Source: CAD feature listing. Evaluate the final solid. Frame: model axes, mm. Face numbers are marked on the shaded views. A direction names the side the tool comes from. Round coordinates to 2 decimals unless told otherwise and drop trailing zeros. Order: outer loops, then holes, each group sorted by start corner. A loop starts at its lowest first (then second) coordinate and runs counter-clockwise, first axis right, second up. Notation, with made-up numbers: (23, 46) -> (43, 46) arc R14 ccw to (43, 68) -> close; hole circle Ø1 at (-10.75, 49). An arc over 180 degrees is marked (long way). Answer as CSV lines item,"result". Start each with the question number.
(1) Contact query for flat-ended pins moving along their axis: P1, Ø5, axis at y = 141, z = 1, coming from the +X side; P2, Ø1.6, axis at x = 20.5, y = 112, coming from the +Z side; P3, Ø5.5, axis at y = 110, z = 0, coming from the +X side; P4, Ø1.6, axis at x = 21.5, y = 121.5, coming from the -Z side. Output: stop coordinate, or through.
(2) Line query: line 1 along Y through (x, z) = (22.2, 0); line 2 along Y through (x, z) = (21.9, 0); line 3 along Z through (x, y) = (21.8, 110). Output: solid intervals per line, ascending. Write a range as from..to.
(3) Section query A-A (z = 0). Count the separate pieces of the cut face and the enclosed holes in it, plus the area to 3 significant figures.
(4) Section query C-C (y = 154.5). Output: boundary loops of the cut face in (x, z).
(5) Set-up query: the marked faces 1 and 2. Return all of +Z, -Z, +X, -X, +Y, -Y with unobstructed straight access to the full face (end or side cutting, diameter ignored); none if empty.
(6) Section query D-D (z = 37.5). Output: boundary loops of the cut face in (x, y).
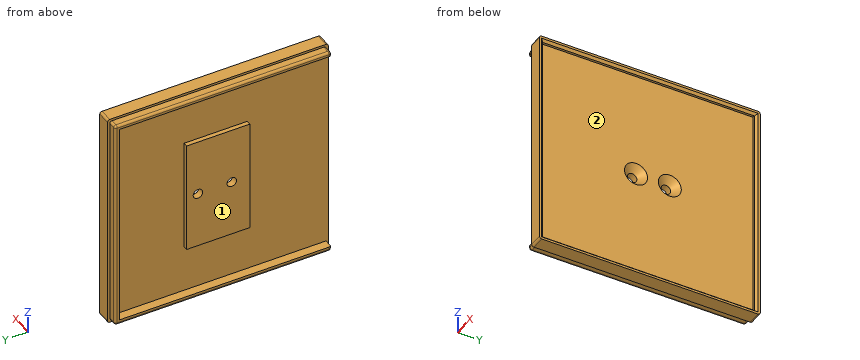
```python
from build123d import *

# Parameters (mm, degrees)
SKETCH009_W     = 98
SKETCH009_H     = 98
PAD006_DEPTH    = 4
SKETCH010_W     = 28
SKETCH010_H     = 50
PAD007_DEPTH    = 2
SKETCH011_R     = 2.1
POCKET003_DEPTH = 6
PAD008_DEPTH    = 4
SKETCH013_W     = 98
SKETCH013_H     = 98
SKETCH013_W_2   = 94
SKETCH013_H_2   = 94
PAD009_DEPTH    = 2
CHAMFER002_SIZE = 3
CHAMFER003_SIZE = 3
CHAMFER004_SIZE = 1
CHAMFER005_SIZE = 1
CHAMFER006_SIZE = 1
CHAMFER007_SIZE = 1
FILLET_R        = 1
FILLET001_R     = 1
FILLET002_R     = 1
FILLET003_R     = 1
FILLET004_R     = 1
FILLET005_R     = 1
FILLET006_R     = 1
FILLET007_R     = 1
FILLET008_R     = 1


with BuildPart() as part:
    # Sketch009 → Pad006 (new body)
    with BuildSketch(Plane.YZ.offset(22)):
        with Locations((115, 0)):
            Rectangle(SKETCH009_W, SKETCH009_H)
    extrude(amount=PAD006_DEPTH)

    # Sketch010 (on Face5 of Pad006) → Pad007 (join)
    with BuildSketch(Plane(origin=(22, 0, 0), x_dir=(0, 1, 0), z_dir=(-1, 0, 0))):
        with Locations((116, 0)):
            Rectangle(SKETCH010_W, SKETCH010_H)
    extrude(amount=PAD007_DEPTH)

    # Sketch011 (on Face11 of Pad007) → Pocket003 (cut)
    with BuildSketch(Plane(origin=(20, 0, 0), x_dir=(0, 1, 0), z_dir=(-1, 0, 0))):
        with Locations((125, 0)):
            Circle(SKETCH011_R)
        with Locations((110, 0)):
            Circle(SKETCH011_R)
    extrude(amount=-POCKET003_DEPTH, mode=Mode.SUBTRACT)

    # Sketch012 (on Face4 of Pocket003) → Pad008 (join)
    with BuildSketch(Plane(origin=(22, 0, 0), x_dir=(0, 1, 0), z_dir=(-1, 0, 0))):
        Polygon((163, 48), (163, -48), (67, -48), (67, -46), (161, -46), (161, 46), (67, 46), (67, 48), align=None)
    extrude(amount=PAD008_DEPTH)

    # Sketch013 (on Face5 of Pad008) → Pad009 (join)
    with BuildSketch(Plane.YZ.offset(26)):
        with Locations((115, 0)):
            Rectangle(SKETCH013_W, SKETCH013_H)
        with Locations((115, 0)):
            Rectangle(SKETCH013_W_2, SKETCH013_H_2, mode=Mode.SUBTRACT)
    extrude(amount=PAD009_DEPTH)

    # Chamfer002
    chamfer002_edges = [part.edges().sort_by_distance(p)[0] for p in [
        (26, 107.9, 0),
    ]]
    chamfer(chamfer002_edges, length=CHAMFER002_SIZE)

    # Chamfer003
    chamfer003_edges = [part.edges().sort_by_distance(p)[0] for p in [
        (26, 122.9, 0),
    ]]
    chamfer(chamfer003_edges, length=CHAMFER003_SIZE)

    # Chamfer004
    chamfer004_edges = [part.edges().sort_by_distance(p)[0] for p in [
        (28, 162, 0),
    ]]
    chamfer(chamfer004_edges, length=CHAMFER004_SIZE)

    # Chamfer005
    chamfer005_edges = [part.edges().sort_by_distance(p)[0] for p in [
        (28, 115, 47),
    ]]
    chamfer(chamfer005_edges, length=CHAMFER005_SIZE)

    # Chamfer006
    chamfer006_edges = [part.edges().sort_by_distance(p)[0] for p in [
        (28, 68, 0.5),
    ]]
    chamfer(chamfer006_edges, length=CHAMFER006_SIZE)

    # Chamfer007
    chamfer007_edges = [part.edges().sort_by_distance(p)[0] for p in [
        (28, 115.5, -47),
    ]]
    chamfer(chamfer007_edges, length=CHAMFER007_SIZE)

    # Fillet
    fillet_edges = [part.edges().sort_by_distance(p)[0] for p in [
        (25, 164, -49),
    ]]
    fillet(fillet_edges, radius=FILLET_R)

    # Fillet001
    fillet001_edges = [part.edges().sort_by_distance(p)[0] for p in [
        (25, 66, -49),
    ]]
    fillet(fillet001_edges, radius=FILLET001_R)

    # Fillet002
    fillet002_edges = [part.edges().sort_by_distance(p)[0] for p in [
        (25, 66, 49),
    ]]
    fillet(fillet002_edges, radius=FILLET002_R)

    # Fillet003
    fillet003_edges = [part.edges().sort_by_distance(p)[0] for p in [
        (25, 164, 49),
    ]]
    fillet(fillet003_edges, radius=FILLET003_R)

    # Fillet004
    fillet004_edges = [part.edges().sort_by_distance(p)[0] for p in [
        (18, 115, -48),
    ]]
    fillet(fillet004_edges, radius=FILLET004_R)

    # Fillet005
    fillet005_edges = [part.edges().sort_by_distance(p)[0] for p in [
        (18, 163, 0.5),
    ]]
    fillet(fillet005_edges, radius=FILLET005_R)

    # Fillet006
    fillet006_edges = [part.edges().sort_by_distance(p)[0] for p in [
        (18, 114.5, 48),
    ]]
    fillet(fillet006_edges, radius=FILLET006_R)

    # Fillet007
    fillet007_edges = [part.edges().sort_by_distance(p)[0] for p in [
        (20.5, 67, -48),
    ]]
    fillet(fillet007_edges, radius=FILLET007_R)

    # Fillet008
    fillet008_edges = [part.edges().sort_by_distance(p)[0] for p in [
        (20.5, 67, 48),
    ]]
    fillet(fillet008_edges, radius=FILLET008_R)


solid = part.part
```
Answer block:
1,P1,"x = 26"
1,P2,"z = 48"
1,P3,"x = 23.65"
1,P4,"z = -49"
2,line 1,"66..107.9, 112.1..122.9, 127.1..164"
2,line 2,"102..107.9, 112.1..122.9, 127.1..130, 161..163"
2,line 3,"-48..-46, -25..-2.1, 2.1..25, 46..48"
3,separate pieces,"3"
3,enclosed holes,"0"
3,area,"394 mm2"
4,outline,"(18, -47) arc R1 ccw to (19, -48) -> (22, -48) -> (22, -49) -> (28, -49) -> (28, -48) -> (27, -47) -> (26, -47) -> (26, 47) -> (27, 47) -> (28, 48) -> (28, 49) -> (22, 49) -> (22, 48) -> (19, 48) arc R1 ccw to (18, 47) -> (18, 46) -> (22, 46) -> (22, -46) -> (18, -46) -> close"
5,face 1,"-X, -Y"
5,face 2,"+X"
6,outline,"(18, 161) -> (22, 161) -> (22, 66) -> (28, 66) -> (28, 67) -> (27, 68) -> (26, 68) -> (26, 162) -> (27, 162) -> (28, 163) -> (28, 164) -> (22, 164) -> (22, 163) -> (19, 163) arc R1 ccw to (18, 162) -> close"
